Can you work these out from the model? Positions are in its coordinate system, mm. A direction names the side the tool comes from. Coordinates: 2 decimals unless noted, no trailing zeros. Loops run counter-clockwise (first coordinate to the right, second up) from the corner with the lowest first, then second, coordinate; pieces in that order, holes last. Notation, with made-up numbers: M -35,-18.75 L 11,-18.75 A21 cw 11,15.25 Z; hole C 87,-26.5 d5. An arc over 180 degrees is marked long. Answer as a JSON object with one key per item and string values. Group by question number.
Item 1: Which directions (+Z, -Z, +X, -X, +Y, -Y) give clear straight access to the entire face, cutting with the end or side of a thin tool? Please do faces 4 (the flat face through (-31, 0, -2.54)), 5 (the cylindrical face through (-32.82, 0.44, 1.11)), 6 (the flat face through (-2.54, -31, -3)).
Item 2: I'm going to push a flat-ended pin straight in: pin 1 Ø4 at (x, y) = (-8, -20.5) entering from -Z. Where does the tip first touch, or does it pass through?
Item 3: Suppose I cut it at A-A (x = 0). Write out the boundary of the cut face in (y, z) (1 decimal).
Item 4: Suppose I cut it at B-B (y = 0). Write out the boundary of the cut face in (x, z) (1 decimal), then the cut area to 3 significant figures.
Item 5: Suppose I cut it at D-D (x = 21). Write out the boundary of the cut face in (y, z) (1 decimal).
Item 6: Suppose I cut it at C-C (z = -5). Write out the boundary of the cut face in (x, y) (1 decimal), then the cut area to 3 significant figures.
Item 7: We'd pull the mould along Y, two halves only. Please class faces 1 (the flat face through (33.274, 0, -3)), 2 (the cylindrical face through (0.44, -32.82, 1.11)), 3 (the flat face through (-2.54, 32, -3)): +Y half, -Y half, draft (parallel to the pull), parting line (faces both ways), or undercut.
Item 8: If I drill on line 1 (Y direction, x = 4, z = -3.5); line 2 (Z direction, x = 0, y = 11.5), over which ranges is the centre line in solid material (lowest first)?
```python
from build123d import *

# Parameters (mm, degrees)
F0_W     = 66.548
F0_H     = 66.548
F0_R     = 11.1125
F1_DEPTH = 1.5875
F2_W     = 66.548
F2_H     = 66.548
F2_W_2   = 64.897
F2_H_2   = 64.897
F3_DEPTH = 6.985
F5_DEPTH = 2.54
F7_DEPTH = 2.54
F8_R     = 1.5875


with BuildPart() as f1:
    # F0 (on Top) → F1 (new body)
    with BuildSketch(Plane.XY):
        Rectangle(F0_W, F0_H)
        Circle(F0_R, mode=Mode.SUBTRACT)
    extrude(amount=F1_DEPTH)

    # F2 (on face) → F3 (join)
    with BuildSketch(Plane(origin=(0, 0, 0), x_dir=(1, 0, 0), z_dir=(0, 0, -1))):
        Rectangle(F2_W, F2_H)
        Rectangle(F2_W_2, F2_H_2, mode=Mode.SUBTRACT)
    extrude(amount=F3_DEPTH)

    # F4 (on Front) → F5 (join, symmetric)
    with BuildSketch(Plane.XZ):
        Polygon((32.4485, -4.1275), (32.4485, -2.54), (29.9085, -2.54), align=None)
        Polygon((-32.512, -4.1275), (-29.972, -2.54), (-32.512, -2.54), align=None)
    extrude(amount=F5_DEPTH, both=True)

    # F6 (on Right) → F7 (join, symmetric)
    with BuildSketch(Plane.YZ):
        Polygon((32.4485, -4.1275), (32.4485, -2.54), (29.9085, -2.54), align=None)
        Polygon((-32.4485, -4.1275), (-29.9085, -2.54), (-32.4485, -2.54), align=None)
    extrude(amount=F7_DEPTH, both=True)

    # F8
    f8_edges = [f1.edges().sort_by_distance(p)[0] for p in [
        (-33.274, 0, 1.5875),
        (0, 33.274, 1.5875),
        (33.274, 0, 1.5875),
        (0, -33.274, 1.5875),
        (-33.274, 33.274, -2.69875),
        (-33.274, -33.274, -2.69875),
        (33.274, -33.274, -2.69875),
        (33.274, 33.274, -2.69875),
    ]]
    fillet(f8_edges, radius=F8_R)


solid = f1.part
```
From the geometry:
{
 "1": {"face 4": "none", "face 5": "+Z, -X, +Y, -Y", "face 6": "-Z"},
 "2": {"pin 1": "z = 0"},
 "3": {"outline": "M -33.3,-7 L -32.4,-7 L -32.4,-4.1 L -29.9,-2.5 L -32.4,-2.5 L -32.4,0 L -11.1,0 L -11.1,1.6 L -31.7,1.6 A1.6 ccw -33.3,0 Z; M 11.1,0 L 32.4,0 L 32.4,-2.5 L 29.9,-2.5 L 32.4,-4.1 L 32.4,-7 L 33.3,-7 L 33.3,0 A1.6 ccw 31.7,1.6 L 11.1,1.6 Z"},
 "4": {"outline": "M -33.3,-7 L -32.4,-7 L -32.4,-4.1 L -30,-2.5 L -32.4,-2.5 L -32.4,0 L -11.1,0 L -11.1,1.6 L -31.7,1.6 A1.6 ccw -33.3,0 Z; M 11.1,0 L 32.4,0 L 32.4,-2.5 L 29.9,-2.5 L 32.4,-4.1 L 32.4,-7 L 33.3,-7 L 33.3,0 A1.6 ccw 31.7,1.6 L 11.1,1.6 Z", "area": "84.7 mm2"},
 "5": {"outline": "M -33.3,-7 L -32.4,-7 L -32.4,0 L 32.4,0 L 32.4,-7 L 33.3,-7 L 33.3,0 A1.6 ccw 31.7,1.6 L -31.7,1.6 A1.6 ccw -33.3,0 Z"},
 "6": {"outline": "M -33.3,-31.7 A1.6 ccw -31.7,-33.3 L 31.7,-33.3 A1.6 ccw 33.3,-31.7 L 33.3,31.7 A1.6 ccw 31.7,33.3 L -31.7,33.3 A1.6 ccw -33.3,31.7 Z; hole M -32.4,-32.4 L 32.4,-32.4 L 32.4,32.4 L -32.4,32.4 Z", "area": "215 mm2"},
 "7": {"face 1": "draft", "face 2": "-Y half", "face 3": "undercut"},
 "8": {"line 1": "-33.27 to -32.45, 32.45 to 33.27", "line 2": "0 to 1.59"}
}
